The figure shows three views and two pictorial views of one solid part (mm, origin at its lowest corner). Answer the questions. A direction names the side the tool comes from. Round coordinates to 2 decimals unless told otherwise and drop trailing zeros. Order: outer loops, then holes, each group sorted by start corner. A loop starts at its lowest first (then second) coordinate and runs counter-clockwise, first axis right, second up. Notation, with made-up numbers: (74.5, 1) -> (97.5, 1) arc R29 cw to (97.5, 23) -> close; hole circle Ø1 at (69.5, 8.5). An arc over 180 degrees is marked (long way). Return JSON: item names as keys, results as strings. Group by question number.
(1) The part is cut by section A-A (x = 3.3). Determine the outline of the cut face in (y, z).
(2) Consider line 1 (Z direction, x = 3.25, y = 7); line 2 (Y direction, x = 5.5, z = 1); line 3 (Y direction, x = 5.5, z = 2). Determine where each line is inside the solid, lowest interval first. Write a range as [from, to].
(3) Which of the six approach directions +Z, -Z, +X, -X, +Y, -Y give full straight-line access (tool end or side, diameter ignored) to the marked faces 1 and 2?
(4) The part is cut by section B-B (z = 3.3). Determine the outline of the cut face in (x, y), plus the area to 3 significant figures.
(5) The part is cut by section C-C (y = 0.5). Determine the outline of the cut face in (x, z).
(6) Each of these flat-tipped pins is pushed along its axis until it touches: pin 1 (1 mm diameter, centred on x = 5, z = 5, fed in from +Y); pin 2 (2 mm diameter, centred on y = 1.5, z = 5.5, fed in from -X); pin 3 (1.5 mm diameter, centred on x = 4.5, y = 8, fed in from +Z). Where does it stop, or does it pass through?
(7) The part is cut by section D-D (y = 7.5). Determine the outline of the cut face in (x, z).
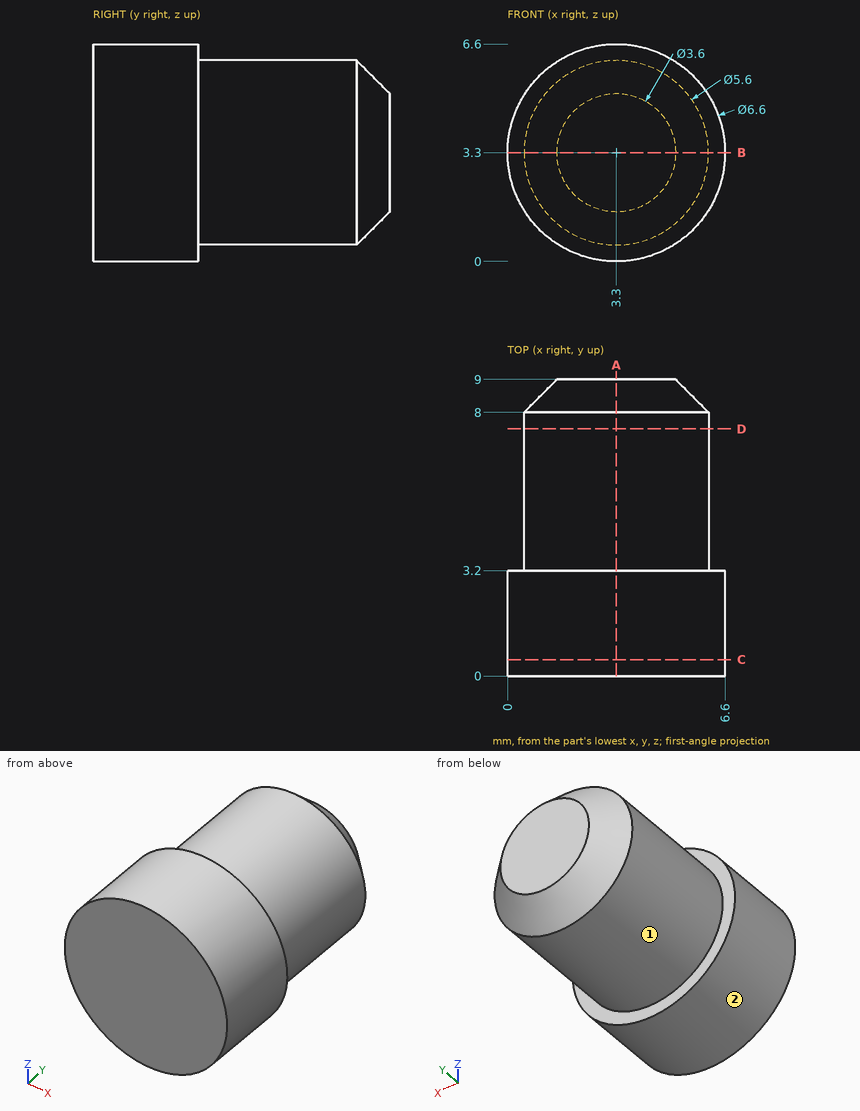
Answer below:
{
 "1": {"outline": "(0, 0) -> (3.2, 0) -> (3.2, 0.5) -> (8, 0.5) -> (9, 1.5) -> (9, 5.1) -> (8, 6.1) -> (3.2, 6.1) -> (3.2, 6.6) -> (0, 6.6) -> close"},
 "2": {"line 1": "z = [0.5, 6.1]", "line 2": "y = [0, 3.2]", "line 3": "y = [0, 8.24]"},
 "3": {"face 1": "+Y", "face 2": "+Y, -Y"},
 "4": {"outline": "(0, 0) -> (6.6, 0) -> (6.6, 3.2) -> (6.1, 3.2) -> (6.1, 8) -> (5.1, 9) -> (1.5, 9) -> (0.5, 8) -> (0.5, 3.2) -> (0, 3.2) -> close", "area": "52.6 mm²"},
 "5": {"outline": "circle Ø6.6 at (3.3, 3.3)"},
 "6": {"pin 1": "stops at y = 8.9", "pin 2": "stops at x = 0.23", "pin 3": "stops at z = 6.06"},
 "7": {"outline": "circle Ø5.6 at (3.3, 3.3)"}
}
